Verification items for this drawing (mm, ordinates from the low corner). Coordinates: 2 decimals unless noted, no trailing zeros. Loops run counter-clockwise (first coordinate to the right, second up) from the corner with the lowest first, then second, coordinate; pieces in that order, holes last. Notation, with made-up numbers: (15, -8) -> (31, -8) arc R15 cw to (31, -4) -> close; hole circle Ø9 at (37.25, -22). An arc over 180 degrees is marked (long way). Write item = value, one per line.
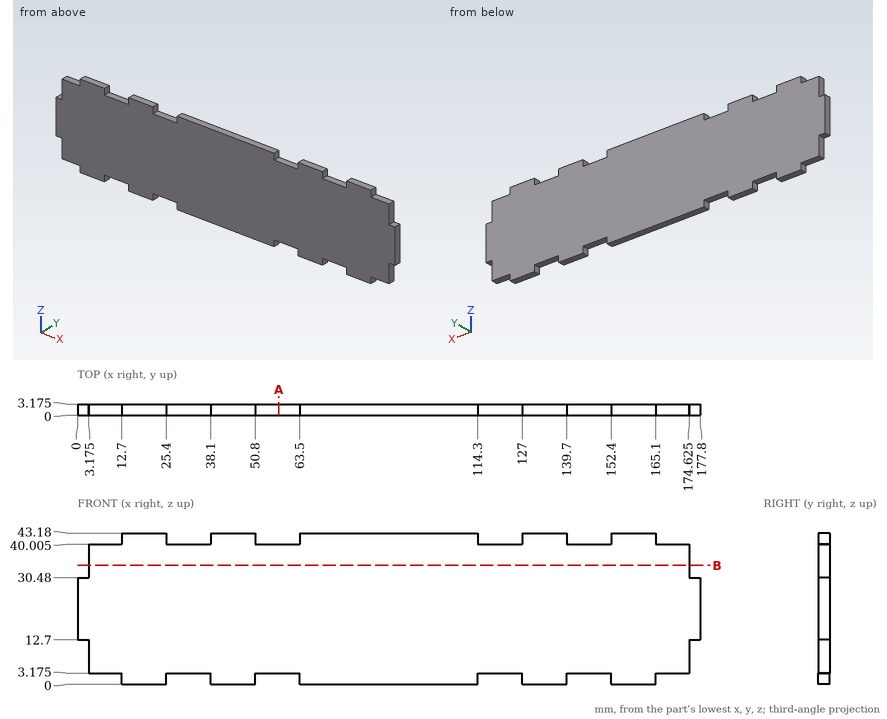
1) Depth check by flat-ended pin: pin 1 Ø1 at (y, z) = (1, 41.5) entering from -X; pin 2 Ø1 at (y, z) = (1.5, 7.5) entering from +X (3 decimals); pin 3 Ø1.6 at (x, y) = (33.5, 1.5) entering from +Z (3 decimals). Enter the tip coordinate at first touch or a pass-through.
Ans:
pin_1 = 12.7
pin_2 = 174.625
pin_3 = 40.005
2) Sectioned sample at A-A, the plane x = 57.5. Record the cut outline in (y, z) (3 decimals), plus the area to 3 significant figures.
Ans:
outline = (0, 3.175) -> (3.175, 3.175) -> (3.175, 40.005) -> (0, 40.005) -> close
area = 117 mm2
3) Sectioned sample at B-B, the plane z = 34. Record the cut outline in (x, y) (3 decimals), plus the area to 3 significant figures.
Ans:
outline = (3.175, 0) -> (174.625, 0) -> (174.625, 3.175) -> (3.175, 3.175) -> close
area = 544 mm2
4) Material ranges on line 1 (X direction, y = 2.95, z = 2); line 2 (X direction, y = 3, z = 4) (3 decimals); line 3 (Z direction, x = 35.5, y = 0.4) (3 decimals), recorded low to high.
Ans:
line_1 = 12.7 to 25.4, 38.1 to 50.8, 63.5 to 114.3, 127 to 139.7, 152.4 to 165.1
line_2 = 3.175 to 174.625
line_3 = 3.175 to 40.005
